```python
from build123d import *

# Parameters (mm, degrees)
F0_W      = 55
F0_H      = 90
F1_DEPTH  = 1.6
F2_W      = 55
F2_H      = 22
F3_DEPTH  = 22
F4_W      = 15
F4_H      = 10
F4_W_2    = 12
F5_DEPTH  = 40
F6_DEPTH  = 7
F7_W      = 9.4927671924
F7_H      = 68
F8_DEPTH  = 2
F9_W      = 10
F9_H      = 8.6
F10_DEPTH = 20
F11_W     = 10
F11_H     = 8.6
F12_DEPTH = 15


with BuildPart() as f1:
    # F0 (on Top) → F1 (new body)
    with BuildSketch(Plane.XY):
        with Locations((-1.4253398404, 6.9053554087)):
            Rectangle(F0_W, F0_H)
    extrude(amount=F1_DEPTH)

    # F2 (on face) → F3 (join)
    with BuildSketch(Plane.XY.offset(1.6)):
        with Locations((-1.4253398404, -27.0946445913)):
            Rectangle(F2_W, F2_H)
    extrude(amount=F3_DEPTH)

    # F4 (on face) → F5 (join)
    with BuildSketch(Plane.XZ.offset(38.0946445913)):
        with Locations((3.5746601596, 15.4229834428)):
            Rectangle(F4_W, F4_H)
        with Locations((-19.0744694758, 15.4229834428)):
            Rectangle(F4_W_2, F4_H)
    extrude(amount=F5_DEPTH)

    # F6 (add): a face of the model
    f6_faces = [f1.faces().sort_by_distance(p)[0] for p in [
        (-1.4253398404, 17.9053554087, 1.6),
    ]]
    extrude(f6_faces, amount=F6_DEPTH)

    # F7 (on face) → F8 (join)
    with BuildSketch(Plane.XY.offset(8.6)):
        with Locations((21.3282765634, 17.9053554087)):
            Rectangle(F7_W, F7_H)
    extrude(amount=F8_DEPTH)

    # F9 (on face) → F10 (join)
    with BuildSketch(Plane(origin=(-28.9253398404, 0, 0), x_dir=(0, -1, 0), z_dir=(-1, 0, 0))):
        with Locations((-38.9053554087, 4.3)):
            Rectangle(F9_W, F9_H)
    extrude(amount=F10_DEPTH)

    # F11 (on face) → F12 (join)
    with BuildSketch(Plane.XZ.offset(-33.9053554087)):
        with Locations((-43.9253398404, 4.3)):
            Rectangle(F11_W, F11_H)
    extrude(amount=F12_DEPTH)


solid = f1.part
```
The model under review builds one solid part; all positions refer to its coordinate system, in mm. A direction names the side the tool comes from. Give positions to 0.01 mm unless a question says otherwise; leave off trailing zeros. Write each loop counter-clockwise with the first axis right and the second up, starting at its lowest first coordinate (ties: lowest second). Pieces come first, ordered by that corner, then holes. Notation, with made-up numbers: (15, -31.75) - (64, -31.75) arc R13 cw to (64, -17.75) - close; hole circle Ø4 at (39.25, -34.5). An arc over 180 degrees is marked (long way). Answer in a Markdown table with one row per item. Add a question column.
1. Tool access review of faces 5 (the flat face through (-9, 18, 8.6)), 6 (the flat face through (-28.925, -11, 6)), 7 (the flat face through (-39, 43.905, 4)): name each direction out of +Z, -Z, +X, -X, +Y, -Y from which nothing blocks a thin tool from reaching the whole face with its end or side.
2. Wall thickness on line 1 along Y through (x, z) = (21, 6.5); line 2 along X through (y, z) = (32, 6.25); line 3 along X through (y, z) = (-25.5, 10): over which ranges is each line inside the solid? List them lowest first. Write a range as [from, to].
3. Draft analysis for pull direction X (two halves, no side actions). For faces 1 (the flat face through (-28.925, 48, 4)), 2 (the flat face through (-13.074, -58, 15)), 3 (the flat face through (26.075, -4, 6)), 4 (the flat face through (3, -58, 20.423)), state which applies: +X half, -X half, draft (parallel to the pull), parting line (faces both ways), or undercut.
4. We need section D-D on y = -51.5. Write out the cut boundary in (x, z), then the cut area to 3 significant figures.
5. Insertion check: P1, Ø7, axis at x = -41.5, z = 3.5, coming from the +Y side; P2, Ø7, axis at y = 15, z = 7, coming from the -X side; P3, Ø5, axis at y = -61.5, z = 14.5, coming from the -X side; P4, Ø12, axis at x = -3, z = 13, coming from the +Y side. Each pin has a flat end and moves straight along its axis. Give the tip position at first contact, or say it passes through.
6. We need section C-C on x = -15. Write out the cut boundary in (y, z), then the cut area to 3 significant figures.
7. We need section A-A on y = 32.5. Write out the cut boundary in (x, z).
8. We need section B-B on z = 12.25. Write out the cut boundary in (x, y).
Ans:
| question | item | result |
|---|---|---|
| 1 | face 5 | +Z, -X, +Y |
| 1 | face 6 | +Z, -Z, -Y |
| 1 | face 7 | +Z, -Z, -X, +Y |
| 2 | line 1 | y = [-38.09, 51.91] |
| 2 | line 2 | x = [-48.93, -38.93], [-28.93, 26.07] |
| 2 | line 3 | x = [-28.93, 26.07] |
| 3 | face 1 | -X half |
| 3 | face 2 | undercut |
| 3 | face 3 | +X half |
| 3 | face 4 | draft |
| 4 | outline | (-25.07, 10.42) - (-13.07, 10.42) - (-13.07, 20.42) - (-25.07, 20.42) - close; (-3.93, 10.42) - (11.07, 10.42) - (11.07, 20.42) - (-3.93, 20.42) - close |
| 4 | area | 270 mm^2 |
| 5 | P1 | stops at y = 43.91 |
| 5 | P2 | stops at x = -28.93 |
| 5 | P3 | stops at x = -25.07 |
| 5 | P4 | stops at y = 51.91 |
| 6 | outline | (-78.09, 10.42) - (-38.09, 10.42) - (-38.09, 0) - (51.91, 0) - (51.91, 8.6) - (-16.09, 8.6) - (-16.09, 23.6) - (-38.09, 23.6) - (-38.09, 20.42) - (-78.09, 20.42) - close |
| 6 | area | 1,500 mm^2 |
| 7 | outline | (-48.93, 0) - (-38.93, 0) - (-38.93, 8.6) - (-48.93, 8.6) - close; (-28.93, 0) - (26.07, 0) - (26.07, 10.6) - (16.58, 10.6) - (16.58, 8.6) - (-28.93, 8.6) - close |
| 8 | outline | (-28.93, -38.09) - (-25.07, -38.09) - (-25.07, -78.09) - (-13.07, -78.09) - (-13.07, -38.09) - (-3.93, -38.09) - (-3.93, -78.09) - (11.07, -78.09) - (11.07, -38.09) - (26.07, -38.09) - (26.07, -16.09) - (-28.93, -16.09) - close |
